The listing builds one solid part. Answer for the finished solid, in the listing's coordinates (mm). Give positions to 0.01 mm unless a question says otherwise; leave off trailing zeros. Write each loop counter-clockwise with the first axis right and the second up, starting at its lowest first coordinate (ties: lowest second). Pieces come first, ordered by that corner, then holes. Notation, with made-up numbers: (-36.5, 28) -> (14.5, 28) arc R30 cw to (14.5, 64) -> close; hole circle Ø3 at (64.5, 88). An arc over 180 degrees is marked (long way). One line per question, with ' | ' between items.
from build123d import *

# Parameters (mm, degrees)
BOSS_EXTRUDE1_DEPTH  = 6.35
M4_CLEARANCE_HOLE1_D = 4.5


with BuildPart() as part:
    # Sketch3 → Boss-Extrude1 (new body)
    with BuildSketch(Plane(origin=(0, 0, 0), x_dir=(1, 0, 0), z_dir=(0, 1, 0))):
        with BuildLine():
            Line((-103.762341406, 50.934626006), (3.339213875, 8.410084854))
            ThreePointArc((3.339213875, 8.410084854), (8.88764963, -1.699870765), (0, -9.04875))
            Line((0, -9.04875), (-82.55, -9.04875))
            ThreePointArc((-82.55, -9.04875), (-87.074375, -7.836447372), (-90.386447372, -4.524375))
            Line((-90.386447372, -4.524375), (-114.938002654, 38.000166152))
            ThreePointArc((-114.938002654, 38.000166152), (-113.948550258, 48.440497232), (-103.762341406, 50.934626006))
        make_face()
    extrude(amount=BOSS_EXTRUDE1_DEPTH)

    # M4 Clearance Hole1 (through all)
    with Locations(Plane(origin=(0, 6.35, 0), x_dir=(1, 0, 0), z_dir=(0, 1, 0))):
        with Locations((-107.101555281, 42.524541152), (-82.55, 0), (0, 0)):
            Hole(M4_CLEARANCE_HOLE1_D / 2)


solid = part.part
Item 1: Find section A-A (x = -107). Write down the section's boundary in (y, z), then the cut area to 3 significant figures.
Answers below:
outline: (0, -51.57) -> (6.35, -51.57) -> (6.35, -44.77) -> (0, -44.77) -> close; (0, -40.28) -> (6.35, -40.28) -> (6.35, -24.25) -> (0, -24.25) -> close | area: 145 mm²
Item 2: A flat-ended cylindrical pin translates along its axis: pin 1 (3 mm diameter, centred on x = -97.5, y = 2, fed in from -Z). Find the tip coordinate at first contact, or state that the pin passes through.
Answers below:
pin 1: z = -49.04
Item 3: Find section B-B (z = 0). Write down the section's boundary in (x, y).
Answers below:
outline: (-93, 0) -> (-84.8, 0) -> (-84.8, 6.35) -> (-93, 6.35) -> close; (-80.3, 0) -> (-2.25, 0) -> (-2.25, 6.35) -> (-80.3, 6.35) -> close; (2.25, 0) -> (9.05, 0) -> (9.05, 6.35) -> (2.25, 6.35) -> close
Item 4: Find section C-C (y = 5). Write down the section's boundary in (x, z).
Answers below:
outline: (-114.94, -38) arc R9.05 ccw to (-103.76, -50.93) -> (3.34, -8.41) arc R9.05 ccw to (0, 9.05) -> (-82.55, 9.05) arc R9.05 ccw to (-90.39, 4.52) -> close; hole circle Ø4.5 at (-107.1, -42.52); hole circle Ø4.5 at (-82.55, 0); hole circle Ø4.5 at (0, 0)
Item 5: Determine the mould class of faces 1 (the face through (-87.017, 3.131, 7.869)), 2 (the face through (-50.96, 3.13, -29.97)), 3 (the face through (-84.63, 3.13, 0.86)) for opening direction X: pulls with the +X half, pulls with the -X half, needs draft (parallel to the pull), parting line crosses it, or undercut.
Answers below:
face 1: pulls with the -X half | face 2: pulls with the +X half | face 3: undercut
Item 6: Consider line 1 (Z direction, x = -82.55, y = 2); line 2 (Z direction, x = -81, y = 4); line 3 (Z direction, x = -29, y = 4.75). Determine where each line is inside the solid, lowest interval first. Write a range as [from, to].
Answers below:
line 1: [-42.51, -2.25], [2.25, 9.05] | line 2: [-41.9, -1.63], [1.63, 9.05] | line 3: [-21.25, 9.05]
Item 7: Find section D-D (x = -23.5). Write down the section's boundary in (y, z).
Answers below:
outline: (0, -19.07) -> (6.35, -19.07) -> (6.35, 9.05) -> (0, 9.05) -> close
